from build123d import *

# Parameters (mm, degrees)
EXTRUSION1_DEPTH = 8
ESQUISSE2_R      = 1.5
EXTRUSION2_DEPTH = 80
ESQUISSE3_R      = 1.5
EXTRUSION3_DEPTH = 80


with BuildPart() as part:
    # Esquisse1 → Extrusion1 (new body)
    with BuildSketch(Plane.XY):
        Polygon((-3.463711982, -6.095820103), (-1.963711982, -6.095820103), (-1.963711982, -19.595820103), (11.536288018, -19.595820103), (11.536288018, -21.095820103), (-3.463711982, -21.095820103), align=None)
    extrude(amount=EXTRUSION1_DEPTH)

    # Esquisse2 → Extrusion2 (cut)
    with BuildSketch(Plane(origin=(-1.963711982, 0, 0), x_dir=(0, 0, -1), z_dir=(1, 0, 0))):
        with Locations(Location((-4, -12.095820103, 0), (0, 0, 90))):
            Circle(ESQUISSE2_R)
    extrude(amount=-EXTRUSION2_DEPTH, mode=Mode.SUBTRACT)

    # Esquisse3 → Extrusion3 (cut)
    with BuildSketch(Plane(origin=(0, -19.595820103, 0), x_dir=(-1, 0, 0), z_dir=(0, 1, 0))):
        with Locations(Location((-5.536288018, 4, 0), (0, 0, 90))):
            Circle(ESQUISSE3_R)
    extrude(amount=-EXTRUSION3_DEPTH, mode=Mode.SUBTRACT)


solid = part.part
Read the model definition and answer for the solid it produces. Units are mm, in the model's axes. A direction names the side the tool comes from. Round coordinates to 2 decimals unless told otherwise and drop trailing zeros. Order: outer loops, then holes, each group sorted by start corner. A loop starts at its lowest first (then second) coordinate and runs counter-clockwise, first axis right, second up. Notation, with made-up numbers: (13.25, -14) - (19.25, -14) arc R19 cw to (19.25, 19) - close; hole circle Ø7 at (45, 23). An arc over 180 degrees is marked (long way). Use one line per item in the form item = value. Start each with the question number.
(1) The part is cut by section D-D (z = 0.75). Give the vertices of the cut face in (x, y).
(2) The part is cut by section A-A (z = 4). Give the vertices of the cut face in (x, y), then the cut area to 4 significant figures.
(3) Find the intervals of material crossed by line 1 along X through (y, z) = (-20.25, 4); line 2 along X through (y, z) = (-14, 1); line 3 along Y through (x, z) = (9.25, 7.5), in increasing order. Write a range as from..to.
(4) The part is cut by section B-B (x = -2.25). Give the vertices of the cut face in (y, z).
(5) For faces 1 (the face through (-3.464, -14, 4)), 2 (the face through (3, -19.596, 4)), determine the directions among +Z, -Z, +X, -X, +Y, -Y from which every point of the face is accessible in a straight line to the end or side of a thin tool.
(6) Flat-ended cylindrical pins translate along their axes: pin 1 Ø2.5 at (y, z) = (-13, 3) entering from +X; pin 2 Ø4 at (x, z) = (8.5, 5) entering from +Y. Find the tip coordinate at first contact, or state that the pin passes through.
(7) The part is cut by section C-C (y = -11). Give the vertices of the cut face in (x, z), then the cut area to 3 significant figures.
(8) Determine the mould class of faces 3 (the face through (1, -20, 0)), 4 (the face through (1, -20, 8)), 5 (the face through (-2.703, -10.665, 4.451)) for opening direction Z: +Z half, -Z half, draft (parallel to the pull), parting line (faces both ways), or undercut.
Checked values:
q1.outline = (-3.46, -21.1) - (11.54, -21.1) - (11.54, -19.6) - (-1.96, -19.6) - (-1.96, -6.1) - (-3.46, -6.1) - close
q2.outline = (-3.46, -21.1) - (4.04, -21.1) - (4.04, -19.6) - (-1.96, -19.6) - (-1.96, -13.6) - (-3.46, -13.6) - close; (-3.46, -10.6) - (-1.96, -10.6) - (-1.96, -6.1) - (-3.46, -6.1) - close; (7.04, -21.1) - (11.54, -21.1) - (11.54, -19.6) - (7.04, -19.6) - close
q2.area = 33.75 mm^2
q3.line_1 = -3.46..4.04, 7.04..11.54
q3.line_2 = -3.46..-1.96
q3.line_3 = -21.1..-19.6
q4.outline = (-21.1, 0) - (-6.1, 0) - (-6.1, 8) - (-21.1, 8) - close; hole circle Ø3 at (-12.1, 4)
q5.face_1 = +Z, -Z, -X, +Y, -Y
q5.face_2 = +Z, -Z, +X, +Y
q6.pin_1 = -1.96
q6.pin_2 = -19.6
q7.outline = (-3.46, 0) - (-1.96, 0) - (-1.96, 2.98) - (-3.46, 2.98) - close; (-3.46, 5.02) - (-1.96, 5.02) - (-1.96, 8) - (-3.46, 8) - close
q7.area = 8.93 mm^2
q8.face_3 = -Z half
q8.face_4 = +Z half
q8.face_5 = undercut
